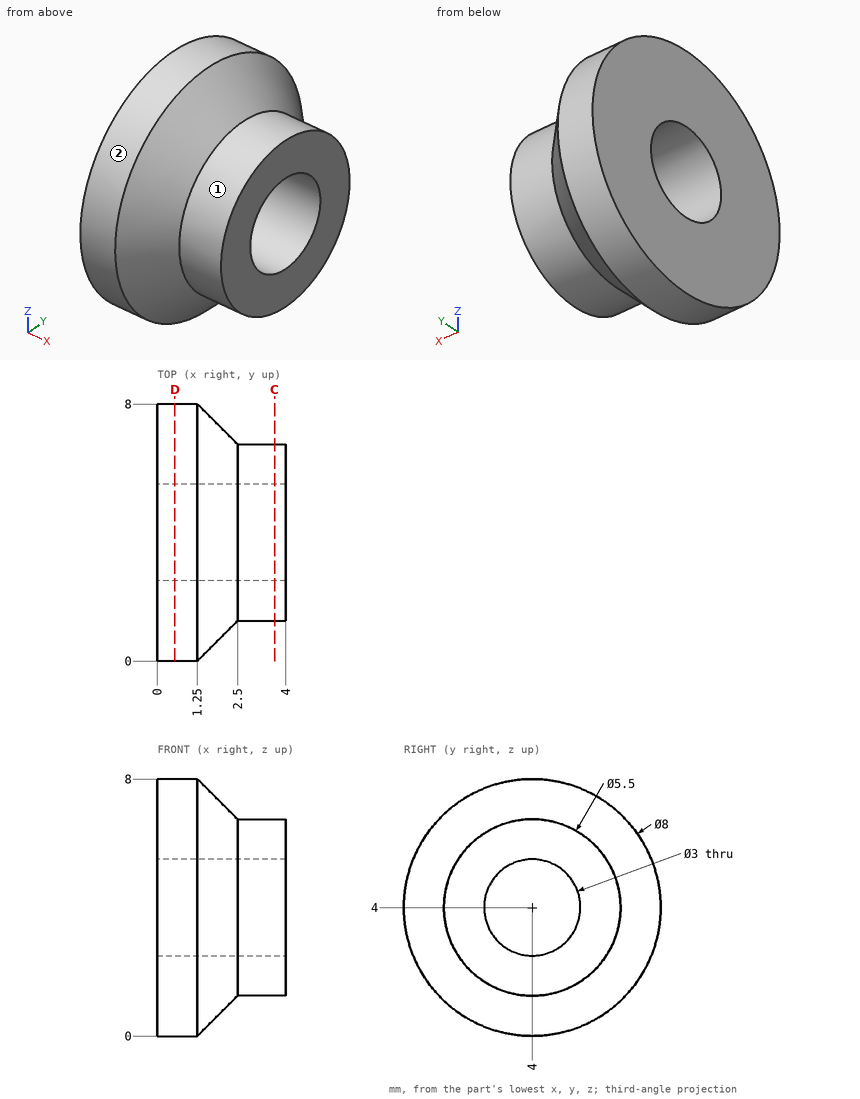
Print and shaded views of the part. All mm, measured from the part's lowest x, y and z. A direction names the side the tool comes from. Coordinates: 2 decimals unless noted, no trailing zeros. Loops run counter-clockwise (first coordinate to the right, second up) from the corner with the lowest first, then second, coordinate; pieces in that order, holes last. Notation, with made-up numbers: M 71,10 L 95,10 A14 cw 95,27 Z; hole C 12,-28 d1. An arc over 180 degrees is marked long. Use a Markdown table: item, result. Add a question column.
Q1. Pin check, flat tips, straight feed: P1, Ø1.7, axis at y = 5, z = 3.5, coming from the +X side; P2, Ø2, axis at x = 0.5, y = 1.5, coming from the +Z side; P3, Ø2, axis at x = 3, z = 6.5, coming from the +Y side; P4, Ø1.5, axis at x = 1, z = 2, coming from the -Y side. Stop position of each tip, or through.
Q2. Cut at D-D (x = 0.55). Write the cut outline in (y, z), and give its area (3 significant figures).
Q3. Which spindle directions (+Z, -Z, +X, -X, +Y, -Y) get a long thin tool onto all of the face, cutting with end or side? Do the marked faces 1 and 2. Say none if no direction does.
Q4. Probe L1, parallel to Y at x = 1.2, z = 4; L2, parallel to Y at x = 3, z = 4; L3, parallel to Z at x = 0.75, y = 3.25. List the from-to ranges inside material, lowest first.
Q5. Cut at C-C (x = 3.65). Write the cut outline in (y, z).
Worked out:
| question | item | result |
|---|---|---|
| 1 | P1 | stops at x = 4 |
| 1 | P2 | stops at z = 7.71 |
| 1 | P3 | stops at y = 6.39 |
| 1 | P4 | stops at y = 0.2 |
| 2 | outline | C 4,4 d8; hole C 4,4 d3 |
| 2 | area | 43.2 mm2 |
| 3 | face 1 | +X |
| 3 | face 2 | +X, -X |
| 4 | L1 | y = 0 to 2.5, 5.5 to 8 |
| 4 | L2 | y = 1.25 to 2.5, 5.5 to 6.75 |
| 4 | L3 | z = 0.07 to 2.7, 5.3 to 7.93 |
| 5 | outline | C 4,4 d5.5; hole C 4,4 d3 |
